Design review of the part built by this model. Coordinates are the model's own, in mm. Face numbers are marked on the shaded views. A direction names the side the tool comes from. Coordinates: 2 decimals unless noted, no trailing zeros. Loops run counter-clockwise (first coordinate to the right, second up) from the corner with the lowest first, then second, coordinate; pieces in that order, holes last. Notation, with made-up numbers: M 21.25,-12 L 56.25,-12 A15 ccw 56.25,14 Z; hole C -15.5,-16 d8. An arc over 180 degrees is marked long. Write item = value, one per line. Start each with the question number.
```python
from build123d import *

# Parameters (mm, degrees)
F0_R     = 22.5
F1_DEPTH = 75
F3_D     = 6.8
F3_DEPTH = 16.45
F3_TIP   = 2.0429261047
F4_R     = 5.2892002913
F5_DEPTH = 3.175
F6_SIZE2 = 5.1961524227
F6_SIZE  = 3


with BuildPart() as f1:
    # F0 (on Front) → F1 (new body)
    with BuildSketch(Plane.XZ):
        Circle(F0_R)
    extrude(amount=-F1_DEPTH)

    # F3
    with Locations(Plane.XZ):
        with Locations((0, -14), (14, 0), (0, 14), (-14, 0)):
            Hole(F3_D / 2, depth=F3_DEPTH)
            with Locations((0, 0, -(F3_DEPTH + F3_TIP / 2))):  # 118° drill point
                Cone(0, F3_D / 2, F3_TIP, mode=Mode.SUBTRACT)

    # F4 (on face) → F5 (join)
    with BuildSketch(Plane.XZ):
        Circle(F4_R)
    extrude(amount=F5_DEPTH)

    # F6
    f6_edges = [f1.edges().sort_by_distance(p)[0] for p in [
        (-22.5, 0, 0),
    ]]
    f6_side = f1.faces().sort_by_distance((-21.863604, 0, 0))[0]
    chamfer(f6_edges, length=F6_SIZE, length2=F6_SIZE2, reference=f6_side)


solid = f1.part
```
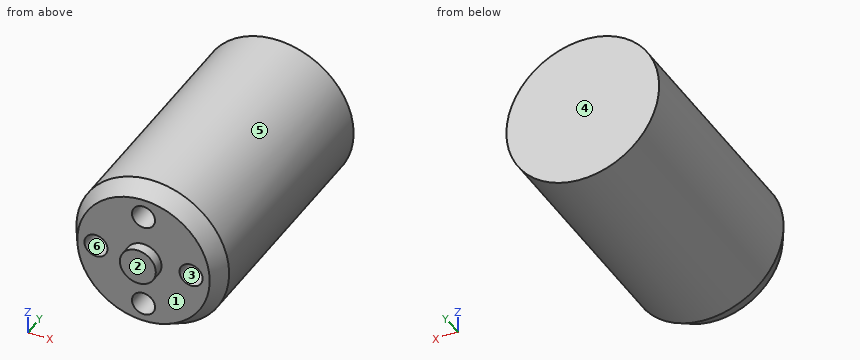
(1) Mouldability with a two-part tool opening along X and no side actions: class the marked faces 3, 4, 5 and 6 as +X half, -X half, draft (parallel to the pull), parting line (faces both ways), or undercut.
(2) To check wall thickness, follow L1, parallel to X at y = 4, z = 0; L2, parallel to Y at x = 16, z = -7.5; L3, parallel to Z at x = -0.5, y = 52.5. State the ranges of each line that lie inside material, in increasing order.
(3) Tool access review of the marked faces 1 and 2: name each direction out of +Z, -Z, +X, -X, +Y, -Y from which nothing blocks a thin tool from reaching the whole face with its end or side.
(4) Insertion check: pin 1 (1.5 mm diameter, centred on x = 11.5, y = 31, fed in from -Z); pin 2 (1 mm diameter, centred on x = 5.5, z = -15, fed in from -Y); pin 3 (8 mm diameter, centred on y = 18.5, z = -8, fed in from -X). Each pin has a flat end and moves straight along its axis. Give the tip position at first contact, or say it passes through.
(5) Take a section at A-A (y = 29.5). State the section outline as (x, z) points, plus the area to 3 significant figures.
Results list:
q1.face_3 = undercut
q1.face_4 = draft
q1.face_5 = parting line
q1.face_6 = undercut
q2.L1 = -21.81 to -17.4, -10.6 to 10.6, 17.4 to 21.81
q2.L2 = 0 to 75
q2.L3 = -22.49 to 22.49
q3.face_1 = -Y
q3.face_2 = +Z, -Z, +X, -X, -Y
q4.pin_1 = -19.77
q4.pin_2 = 0
q4.pin_3 = -22.14
q5.outline = C 0,0 d45
q5.area = 1,590 mm^2
